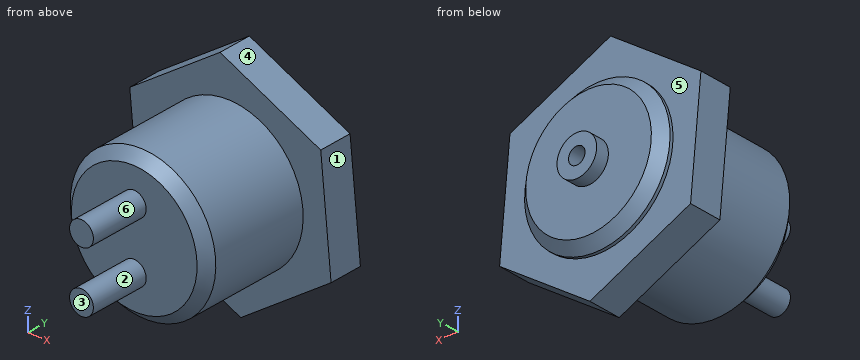
from build123d import *

# Parameters (mm, degrees)
SKETCH_1_R             = 11
EXTRUDE_1_DEPTH        = 23.4
SKETCH_2_R             = 3
EXTRUDE_2_DEPTH        = 2
HOLE_WIZARD_M3_1_D     = 2.5
HOLE_WIZARD_M3_1_DEPTH = 7.5
HOLE_WIZARD_M3_1_TIP   = 0.751075774
CHAMFER_1_SIZE         = 1.5
CHAMFER_2_SIZE         = 1.5
SKETCH_5_R             = 1.8
EXTRUDE_3_DEPTH        = 9
EXTRUDE_4_DEPTH        = 5


with BuildPart() as part:
    # 草图1 → 凸台-拉伸1 (new body)
    with BuildSketch(Plane(origin=(0, 0, 0), x_dir=(1, 0, 0), z_dir=(0, 1, 0))):
        with Locations(Location((0, 0, 0), (0, 0, 270))):
            Circle(SKETCH_1_R)
    extrude(amount=EXTRUDE_1_DEPTH)

    # 草图2 → 凸台-拉伸2 (add)
    with BuildSketch(Plane(origin=(0, 23.4, 0), x_dir=(1, 0, 0), z_dir=(0, 1, 0))):
        with Locations(Location((0, 0, 0), (0, 0, 270))):
            Circle(SKETCH_2_R)
    extrude(amount=EXTRUDE_2_DEPTH)

    # M3 螺纹孔1
    with Locations(Plane(origin=(0, 25.4, 0), x_dir=(-1, 0, 0), z_dir=(0, 1, 0))):
        with Locations((0, 0)):
            Hole(HOLE_WIZARD_M3_1_D / 2, depth=HOLE_WIZARD_M3_1_DEPTH)
            with Locations((0, 0, -(HOLE_WIZARD_M3_1_DEPTH + HOLE_WIZARD_M3_1_TIP / 2))):  # 118° drill point
                Cone(0, HOLE_WIZARD_M3_1_D / 2, HOLE_WIZARD_M3_1_TIP, mode=Mode.SUBTRACT)

    # 倒角1
    chamfer_1_edges = [part.edges().sort_by_distance(p)[0] for p in [
        (0, 23.4, -11),
    ]]
    chamfer(chamfer_1_edges, length=CHAMFER_1_SIZE)

    # 倒角2
    chamfer_2_edges = [part.edges().sort_by_distance(p)[0] for p in [
        (0, 0, -11),
    ]]
    chamfer(chamfer_2_edges, length=CHAMFER_2_SIZE)

    # 草图5 → 凸台-拉伸3 (add)
    with BuildSketch(Plane.XZ):
        with Locations(Location((0, 4.5, 0), (0, 0, 90))):
            Circle(SKETCH_5_R)
        with Locations(Location((0, -4.5, 0), (0, 0, 90))):
            Circle(SKETCH_5_R)
    extrude(amount=EXTRUDE_3_DEPTH)

    # 草图6 → 凸台-拉伸4 (add)
    with BuildSketch(Plane(origin=(0, 16.4, 0), x_dir=(-1, 0, 0), z_dir=(0, 1, 0))):
        Polygon((13.652715142, -9.69209485), (15.219957927, 6.977550719), (1.567242785, 16.669645569), (-13.652715142, 9.69209485), (-15.219957927, -6.977550719), (-1.567242785, -16.669645569), align=None)
    extrude(amount=EXTRUDE_4_DEPTH)


solid = part.part
Verification items for the finished model (mm, model axes). Face numbers are marked on the shaded views. A direction names the side the tool comes from. Round coordinates to 2 decimals unless told otherwise and drop trailing zeros. Loops run counter-clockwise (first coordinate to the right, second up) from the corner with the lowest first, then second, coordinate; pieces in that order, holes last. Notation, with made-up numbers: (41, 29) - (48, 29) arc R23 ccw to (48, 45) - close; hole circle Ø6 at (-34.5, 66). An arc over 180 degrees is marked (long way). Use one line per item in the form item = value.
1. Section check D-D on z = -14. Record the cut outline in (x, y).
A:
outline = (-4.26, 16.4) - (5.33, 16.4) - (5.33, 21.4) - (-4.26, 21.4) - close
2. Access from +Z, -Z, +X, -X, +Y, -Y to the whole of each face (thin tool, end or side, straight path). Record for the marked faces 4, 5 and 6.
A:
face_4 = +Z, +X, +Y, -Y
face_5 = +Y
face_6 = -Y
3. Section check C-C on x = -12. Record the cut outline in (y, z), and give its area (3 significant figures).
A:
outline = (16.4, -10.45) - (21.4, -10.45) - (21.4, 9.26) - (16.4, 9.26) - close
area = 98.6 mm²
4. Scan lines: probe 1 along Z at (x, y) = (-8.5, 13); probe 2 along Y at (x, z) = (-9, -1.5); probe 3 along Z at (x, y) = (0, 22.95). Record each from-to range of solid material in increasing order.
A:
probe_1 = -6.98 to 6.98
probe_2 = 0 to 23.4
probe_3 = -9.95 to -1.25, 1.25 to 9.95
5. Section check B-B on y = 10. Record the cut outline in (x, z), and give its area (3 significant figures).
A:
outline = circle Ø22 at (0, 0)
area = 380 mm²
6. Gauge pin test, flat ends, axial feed: pin 1 Ø15 at (x, z) = (3, -1) entering from +Y; pin 2 Ø4 at (x, y) = (-3, -4) entering from +Z; pin 3 Ø12 at (y, z) = (0.5, -7.5) entering from +X; pin 4 Ø5 at (x, z) = (8.5, -0.5) entering from +Y. Record the tip position at first contact, or that the pin passes through.
A:
pin_1 = 25.4
pin_2 = 6
pin_3 = 10.89
pin_4 = 23.4
7. Draft check along Z on the marked faces 1, 2 and 3. Enter one of: pulls with the +Z half, pulls with the -Z half, needs draft (parallel to the pull), parting line crosses it, or undercut.
A:
face_1 = pulls with the +Z half
face_2 = undercut
face_3 = needs draft
8. Section check A-A on z = 0. Record the cut outline in (x, y), and give its area (3 significant figures).
A:
outline = (-14.56, 16.4) - (-11, 16.4) - (-11, 1.5) - (-9.5, 0) - (9.5, 0) - (11, 1.5) - (11, 16.4) - (14.56, 16.4) - (14.56, 21.4) - (11, 21.4) - (11, 21.9) - (9.5, 23.4) - (3, 23.4) - (3, 25.4) - (1.25, 25.4) - (1.25, 21.4) - (-1.25, 21.4) - (-1.25, 25.4) - (-3, 25.4) - (-3, 23.4) - (-9.5, 23.4) - (-11, 21.9) - (-11, 21.4) - (-14.56, 21.4) - close
area = 548 mm²
